Autodesk Inventor part; units mm, degrees
ref_plane "YZ Plane" through (0, 0, 0) normal (1, 0, 0) x (0, 1, 0)
ref_plane "XZ Plane" through (0, 0, 0) normal (0, 1, 0) x (-1, 0, 0)
ref_plane "XY Plane" through (0, 0, 0) normal (0, 0, 1) x (1, 0, 0)
sketch "Sketch1" plane through (0, 0, 0) normal (0, 0, 1) x (1, 0, 0)
  line L0 (-30, 17.5) -> (30, 17.5)
  line L1 (30, 17.5) -> (30, -17.5)
  line L2 (30, -17.5) -> (-30, -17.5)
  line L3 (-30, -17.5) -> (-30, 17.5)
  point P0 (0, 0)
  point P1 (0, 17.5)
  point P2 (-30, 0)
  dimension "d0" = 60
  dimension "d1" = 35
extrude "Extrusion1" add sketch "Sketch1" along normal blind 8
sketch "Sketch2" plane through (0, 0, 8) normal (0, 0, 1) x (1, 0, 0)
  line L0 (0, 5) -> (0, 0) construction
  line L1 (-10.5, 5) -> (-10.5, 0)
  line L2 (10.5, 0) -> (10.5, 5)
  arc A0 (10.5, 5) -> (-10.5, 5) centre (0, 5) ccw
  arc A1 (-10.5, 0) -> (10.5, 0) centre (0, 0) ccw
  line L3 (-30, -17.5) -> (30, -17.5)
  line L4 (30, 17.5) -> (-30, 17.5)
  circle A2 centre (0, 2.5) radius 10.5
  point P0 (0, 0)
  point P1 (0, 17.5)
  dimension "d4" = 5
  dimension "d5" = 21
  dimension "d17" = 21
  dimension "d18" = 15
extrude "Extrusion2" cut sketch "Sketch2" against normal through all contours A2
sketch "Sketch3" plane through (0, 0, 8) normal (0, 0, 1) x (1, 0, 0)
  circle A0 centre (25, 5) radius 1.75
  circle A1 centre (25, 15) radius 1.75
  line L0 (30, 17.5) -> (-30, 17.5)
  line L1 (30, -17.5) -> (30, 17.5)
  circle A2 centre (-25, 5) radius 1.75
  circle A3 centre (-25, 15) radius 1.75
  line L2 (-30, 17.5) -> (-30, -17.5)
  point P0 (0, 0)
  dimension "d9" = 3.5
  dimension "d10" = 3.5
  dimension "d11" = 10
  dimension "d12" = 2.5
  dimension "d13" = 5
  dimension "d14" = 5
extrude "Extrusion3" cut sketch "Sketch3" against normal through all contours A0 | A2
move faces "Move1" translate (0, -3, 0) faces at (10, 17.5, 2.6667)
equation "\"d14\" = d13"
properties part number "0005-10-002 Suport1 Seringa"
Can you work these out from the model? Positions are in its coordinate system, mm. Coordinates: 2 decimals unless noted, no trailing zeros. Order: outer loops, then holes, each group sorted by start corner. A loop starts at its lowest first (then second) coordinate and runs counter-clockwise, first axis right, second up.
1. Thinking about a two-plate mould opening in X: for faces 1 (the face through (4.845, -6.815, 4.056)), 2 (the face through (-0.4, -8.4, 0)), 3 (the face through (-30, -2, 4)), which applies, +X half, -X half, draft (parallel to the pull), parting line (faces both ways), or undercut?
2. If we section it at B-B (z = 6): Please give me the cut outline in (x, y), then the cut area to 3 significant figures.
3. If we section it at C-C (y = 12): Please give me the cut outline in (x, z).
4. If we section it at A-A (x = 0): Please give me the cut outline in (y, z), then the cut area to 3 significant figures.
5. I need wall thicknesses on line 1 (Y direction, x = 0, z = 2.75); line 2 (Y direction, x = -25, z = 5.75); line 3 (X direction, y = 4, z = 4). Which ranges of each line are inside material? Lowest first, please.
Entries:
1. face 1: undercut
1. face 2: draft
1. face 3: -X half
2. outline: (-30, -17.5) - (30, -17.5) - (30, 14.5) - (-30, 14.5) - close; hole circle Ø3.5 at (-25, 5); hole circle Ø21 at (0, 2.5); hole circle Ø3.5 at (25, 5)
2. area: 1,550 mm2
3. outline: (-30, 0) - (-4.47, 0) - (-4.47, 8) - (-30, 8) - close; (4.47, 0) - (30, 0) - (30, 8) - (4.47, 8) - close
4. outline: (-17.5, 0) - (-8, 0) - (-8, 8) - (-17.5, 8) - close; (13, 0) - (14.5, 0) - (14.5, 8) - (13, 8) - close
4. area: 88.0 mm2
5. line 1: y = -17.5 to -8, 13 to 14.5
5. line 2: y = -17.5 to 3.25, 6.75 to 14.5
5. line 3: x = -30 to -26.44, -23.56 to -10.39, 10.39 to 23.56, 26.44 to 30
